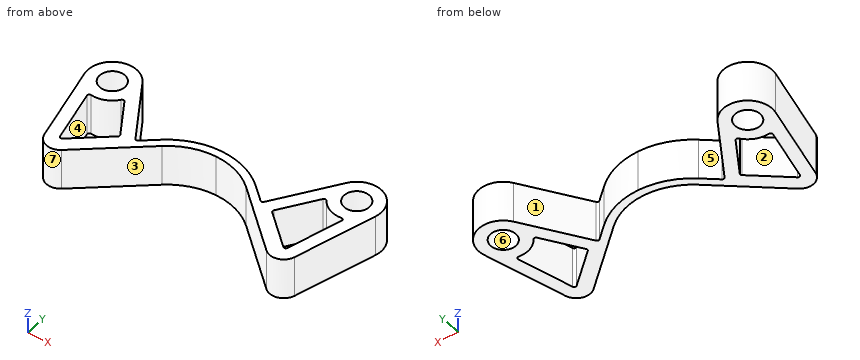
```python
from build123d import *

# Parameters (mm, degrees)
F0_R     = 3.1
F1_DEPTH = 10


with BuildPart() as f1:
    # F0 (on Top) → F1 (new body)
    with BuildSketch(Plane.XY):
        with BuildLine():
            Line((10.5, 10.414885), (25.544604, -2.64322))
            ThreePointArc((25.544604, -2.64322), (28.879034, -3.341846), (31.227885, -0.874176))
            Line((31.227885, -0.874176), (36.30984, 18.827949))
            ThreePointArc((36.30984, 18.827949), (32.905301, 25.823311), (25.456785, 23.577072))
            Line((25.456785, 23.577072), (16.030713, 8.952498))
            ThreePointArc((16.030713, 8.952498), (15.681068, 8.728389), (15.282701, 8.845773))
            Line((15.282701, 8.845773), (11.778201, 11.887536))
            ThreePointArc((11.778201, 11.887536), (6.28637, 15.150615), (0, 16.286148))
            ThreePointArc((0, 16.286148), (-6.28637, 15.150615), (-11.778201, 11.887536))
            Line((-11.778201, 11.887536), (-15.282701, 8.845773))
            ThreePointArc((-15.282701, 8.845773), (-15.681068, 8.728389), (-16.030713, 8.952498))
            Line((-16.030713, 8.952498), (-25.456785, 23.577072))
            ThreePointArc((-25.456785, 23.577072), (-32.905301, 25.823311), (-36.30984, 18.827949))
            Line((-36.30984, 18.827949), (-31.227885, -0.874176))
            ThreePointArc((-31.227885, -0.874176), (-28.879034, -3.341846), (-25.544604, -2.64322))
            Line((-25.544604, -2.64322), (-10.5, 10.414885))
            ThreePointArc((-10.5, 10.414885), (-5.604157, 13.323846), (0, 14.336148))
            ThreePointArc((0, 14.336148), (5.604157, 13.323846), (10.5, 10.414885))
        make_face()
        with BuildLine():
            Line((-19.258958, 7.446964), (-27.566221, 0.236597))
            ThreePointArc((-27.566221, 0.236597), (-28.042568, 0.136794), (-28.378118, 0.489318))
            Line((-28.378118, 0.489318), (-31.799338, 13.752974))
            ThreePointArc((-31.799338, 13.752974), (-31.69041, 14.208319), (-31.252478, 14.373909))
            ThreePointArc((-31.252478, 14.373909), (-28.094699, 14.829762), (-25.617044, 16.839884))
            ThreePointArc((-25.617044, 16.839884), (-25.198241, 17.049189), (-24.789863, 16.820208))
            Line((-24.789863, 16.820208), (-19.166434, 8.095445))
            ThreePointArc((-19.166434, 8.095445), (-19.091715, 7.753943), (-19.258958, 7.446964))
        make_face(mode=Mode.SUBTRACT)
        with BuildLine():
            ThreePointArc((24.789863, 16.820208), (25.198241, 17.049189), (25.617044, 16.839884))
            ThreePointArc((25.617044, 16.839884), (28.094699, 14.829762), (31.252478, 14.373909))
            ThreePointArc((31.252478, 14.373909), (31.69041, 14.208319), (31.799338, 13.752974))
            Line((31.799338, 13.752974), (28.378118, 0.489318))
            ThreePointArc((28.378118, 0.489318), (28.042568, 0.136794), (27.566221, 0.236597))
            Line((27.566221, 0.236597), (19.258958, 7.446964))
            ThreePointArc((19.258958, 7.446964), (19.091715, 7.753943), (19.166434, 8.095445))
            Line((19.166434, 8.095445), (24.789863, 16.820208))
        make_face(mode=Mode.SUBTRACT)
        with Locations((-30.5, 20.326536)):
            Circle(F0_R, mode=Mode.SUBTRACT)
        with Locations((30.5, 20.326536)):
            Circle(F0_R, mode=Mode.SUBTRACT)
    extrude(amount=F1_DEPTH)


solid = f1.part
```
CAD build for the part. Positions are in the model's coordinates, mm. Face numbers are marked on the shaded views. A direction names the side the tool comes from. Round coordinates to 2 decimals unless told otherwise and drop trailing zeros. Write each loop counter-clockwise with the first axis right and the second up, starting at its lowest first coordinate (ties: lowest second). Pieces come first, ordered by that corner, then holes. Notation, with made-up numbers: (85.25, -11.5) - (100.25, -11.5) arc R17 ccw to (100.25, 12.5) - close; hole circle Ø10 at (53, 62). An arc over 180 degrees is marked (long way). Write item = value, one per line. Start each with the question number.
Q1. Band-saw the part on C-C (y = 1.25). Give the cut face in (x, z), then the cut area to 3 significant figures.
Q2. Which spindle directions (+Z, -Z, +X, -X, +Y, -Y) get a long thin tool onto all of the face, cutting with end or side? Do the marked faces 1, 2 and 3. Say none if no direction does.
Q3. Probe L1, parallel to X at y = 4, z = 6; L2, parallel to X at y = 19.5, z = 2; L3, parallel to X at y = 11, z = 1. List the from-to ranges inside material, lowest first. Write a range as from..to.
Q4. Mould opens along Y. For the marked faces 4, 5, 6 and 7 say: pulls with the +Y half, pulls with the -Y half, needs draft (parallel to the pull), parting line crosses it, or undercut.
Q5. Drop flat-ended pins along their axis: pin 1 (5 mm diameter, centred on x = -23.5, z = 2, fed in from -Y); pin 2 (1.5 mm diameter, centred on y = 0.5, z = 3.5, fed in from -X). Give the stop position or say it passes through.
Q6. Band-saw the part on B-B (y = 24.25). Give the cut face in (x, z), then the cut area to 3 significant figures.
Q7. Band-saw the part on A-A (x = 23.5). Give the cut face in (y, z).
Q8. Band-saw the part on D-D (x = -30.5). Give the cut face in (y, z), then the cut area to 3 significant figures.
Answers below:
q1.outline = (-31.78, 0) - (-28.57, 0) - (-28.57, 10) - (-31.78, 10) - close; (-26.4, 0) - (-21.06, 0) - (-21.06, 10) - (-26.4, 10) - close; (21.06, 0) - (26.4, 0) - (26.4, 10) - (21.06, 10) - close; (28.57, 0) - (31.78, 0) - (31.78, 10) - (28.57, 10) - close
q1.area = 171 mm2
q2.face_1 = +Z, -Z, +Y
q2.face_2 = +Z, -Z
q2.face_3 = +Z, -Z, -Y
q3.L1 = -32.49..-29.28, -23.23..-17.89, 17.89..23.23, 29.28..32.49
q3.L2 = -36.44..-33.49, -27.51..-22.83, 22.83..27.51, 33.49..36.44
q3.L3 = -34.29..-31.09, -21.04..-17.35, -12.8..-9.79, 9.79..12.8, 17.35..21.04, 31.09..34.29
q4.face_4 = undercut
q4.face_5 = pulls with the +Y half
q4.face_6 = undercut
q4.face_7 = pulls with the -Y half
q5.pin_1 = -2.98
q5.pin_2 = -31.78
q6.outline = (-35.04, 0) - (-25.96, 0) - (-25.96, 10) - (-35.04, 10) - close; (25.96, 0) - (35.04, 0) - (35.04, 10) - (25.96, 10) - close
q6.area = 182 mm2
q7.outline = (-0.87, 0) - (3.77, 0) - (3.77, 10) - (-0.87, 10) - close; (14.82, 0) - (20.54, 0) - (20.54, 10) - (14.82, 10) - close
q8.outline = (-2.27, 0) - (8.72, 0) - (8.72, 10) - (-2.27, 10) - close; (14.33, 0) - (17.23, 0) - (17.23, 10) - (14.33, 10) - close; (23.43, 0) - (26.33, 0) - (26.33, 10) - (23.43, 10) - close
q8.area = 168 mm2
